Can you work these out from the model? Positions are in its coordinate system, mm. Face numbers are marked on the shaded views. A direction names the side the tool comes from. Round coordinates to 2 decimals unless told otherwise and drop trailing zeros. Write each loop counter-clockwise with the first axis right and the second up, starting at its lowest first coordinate (ties: lowest second). Pieces come first, ordered by that corner, then holes. Notation, with made-up numbers: (-6, -3.5) -> (45, -3.5) arc R24 ccw to (45, 19.5) -> close; hole circle Ø10 at (54, 56). An arc over 180 degrees is marked (long way). Write item = value, one per line. Start each with the question number.
1) For the marked faces 1, 2 and 3, which set-ups out of +Z, -Z, +X, -X, +Y, -Y let a thin tool reach every point of the face, with its end or its side?
2) Imagine slicing it at A-A, the plane z = 50.8. Please give me the cut outline in (x, y), then the cut area to 3 significant figures.
3) If I drill on line 1 (Y direction, x = 7.5, z = 50.8); line 2 (Z direction, x = 50.8, y = -12); line 3 (Y direction, x = 10, z = 52.5), over which ranges is the centre line in solid material (lowest first)?
4) Thinking about a two-plate mould opening in Y: for the marked faces 4, 5, 6 and 7, which applies, +Y half, -Y half, draft (parallel to the pull), parting line (faces both ways), or undercut?
5) Imagine slicing it at B-B, the plane y = -20. Please give me the cut outline in (x, z).
6) I'm going to push flat-ended pins straight in: pin 1 (5 mm diameter, centred on x = 74, z = 24, fed in from -Y); pin 2 (8 mm diameter, centred on x = 16, y = 21, fed in from -Z); pin 3 (1 mm diameter, centred on x = -3, y = -91, fed in from -Z). Where does each tip first touch, or does it pass through?
7) Imagine slicing it at D-D, the plane z = 85. Please give me the cut outline in (x, y), then the cut area to 3 significant figures.
8) Imagine slicing it at C-C, the plane x = 50.8. Please give me the cut outline in (y, z).
from build123d import *

# Parameters (mm, degrees)
F1_DEPTH       = 101.6
F2_R           = 25.4
F4_DEPTH       = 101.6
F3_R           = 25.4
F5_DEPTH       = 101.6
F6_R           = 25.4
F7_DEPTH       = 101.6
F8_R           = 6.35
F10_R          = 25.4
F11_DEPTH      = 50.8
F11_DEPTH_BACK = 152.4


with BuildPart() as f1:
    # F0 (on Front) → F1 (new body)
    with BuildSketch(Plane.XZ):
        Polygon((0, 3.0090576449), (0, 0), (101.6, 0), (101.6, 101.6), (0, 101.6), align=None)
    extrude(amount=F1_DEPTH)

    # F2 (on face) → F4 (cut)
    with BuildSketch(Plane.XY.offset(101.6)):
        with Locations((50.8, -48.6417040229)):
            Circle(F2_R)
    extrude(amount=-F4_DEPTH, mode=Mode.SUBTRACT)

    # F3 (on face) → F5 (cut)
    with BuildSketch(Plane.YZ.offset(101.6)):
        with Locations((-50.8, 50.8)):
            Circle(F3_R)
    extrude(amount=-F5_DEPTH, mode=Mode.SUBTRACT)

    # F6 (on face) → F7 (cut)
    with BuildSketch(Plane(origin=(0, 0, 0), x_dir=(-1, 0, 0), z_dir=(0, 1, 0))):
        with Locations((-50.8, 50.8)):
            Circle(F6_R)
    extrude(amount=-F7_DEPTH, mode=Mode.SUBTRACT)

    # F8
    f8_edges = [f1.edges().sort_by_distance(p)[0] for p in [
        (101.6, -50.8, 0),
        (101.6, -101.6, 50.8),
        (101.6, 0, 50.8),
        (101.6, -50.8, 101.6),
        (50.8, -101.6, 101.6),
        (0, -50.8, 101.6),
        (50.8, 0, 101.6),
        (50.8, -101.6, 0),
        (0, -101.6, 50.8),
        (0, -50.8, 0),
        (0, 0, 50.8),
    ]]
    fillet(f8_edges, radius=F8_R)

    # F10 (on offset) → F11 (join, two sides)
    with BuildSketch(Plane.XZ.offset(101.6)) as f11_sk:
        Circle(F10_R)
    extrude(amount=F11_DEPTH)
    extrude(f11_sk.sketch, amount=-F11_DEPTH_BACK)


solid = f1.part
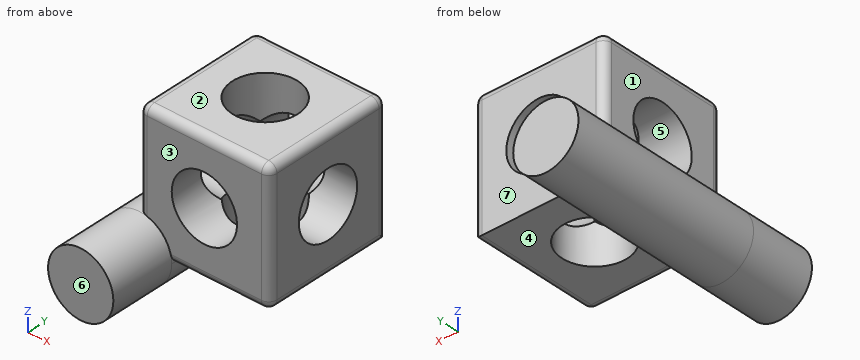
Reported:
q1.face_1 = +Z, -X, +Y, -Y
q1.face_2 = +Z, +X, -X, +Y, -Y
q1.face_3 = +Z, +X, -Y
q2.outline = (0, -95.25) arc R6.35 ccw to (6.35, -101.6) -> (25.4, -101.6) -> (25.4, -76.2) -> (0, -76.2) -> close; (0, -25.4) -> (25.4, -25.4) -> (25.4, 0) -> (6.35, 0) arc R6.35 ccw to (0, -6.35) -> close; (76.2, -101.6) -> (95.25, -101.6) arc R6.35 ccw to (101.6, -95.25) -> (101.6, -76.2) -> (76.2, -76.2) -> close; (76.2, -25.4) -> (101.6, -25.4) -> (101.6, -6.35) arc R6.35 ccw to (95.25, 0) -> (76.2, 0) -> close
q2.area = 2,550 mm²
q3.line_1 = -101.6 to -76.2, -25.4 to 0
q3.line_2 = 0 to 25.4, 76.2 to 101.6
q3.line_3 = -101.6 to -76.14, -25.46 to 0
q4.face_4 = draft
q4.face_5 = undercut
q4.face_6 = -Y half
q4.face_7 = +Y half
q5.outline = (0, 25.4) arc R25.4 ccw (long way) to (25.4, 0) -> (95.25, 0) arc R6.35 ccw to (101.6, 6.35) -> (101.6, 95.25) arc R6.35 ccw to (95.25, 101.6) -> (6.35, 101.6) arc R6.35 ccw to (0, 95.25) -> close; hole circle Ø50.8 at (50.8, 50.8)
q6.pin_1 = -101.6
q6.pin_2 = -22.39
q6.pin_3 = -25.28
q7.outline = (0, -95.25) arc R6.35 ccw to (6.35, -101.6) -> (95.25, -101.6) arc R6.35 ccw to (101.6, -95.25) -> (101.6, -6.35) arc R6.35 ccw to (95.25, 0) -> (6.35, 0) arc R6.35 ccw to (0, -6.35) -> close; hole circle Ø50.8 at (50.8, -48.64)
q7.area = 8,260 mm²
q8.outline = (-101.6, 6.35) arc R6.35 ccw to (-95.25, 0) -> (-74.04, 0) -> (-74.04, 25.4) -> (-101.6, 25.4) -> close; (-101.6, 76.2) -> (-74.04, 76.2) -> (-74.04, 101.6) -> (-95.25, 101.6) arc R6.35 ccw to (-101.6, 95.25) -> close; (-23.24, 0) -> (0, 0) -> (0, 25.4) -> (-23.24, 25.4) -> close; (-23.24, 76.2) -> (0, 76.2) -> (0, 95.25) arc R6.35 ccw to (-6.35, 101.6) -> (-23.24, 101.6) -> close
